Source: three-view drawing plus pictorial views. Frame: mm from the lowest corner of the part. A direction names the side the tool comes from. Give positions to 0.01 mm unless a question says otherwise; leave off trailing zeros. Loops run counter-clockwise (first coordinate to the right, second up) from the corner with the lowest first, then second, coordinate; pieces in that order, holes last. Notation, with made-up numbers: (-15, 6) - (7, 6) arc R29 cw to (7, 32) - close; hole circle Ø10 at (4, 45). An arc over 180 degrees is marked (long way). Put each result on its own line as item: value.
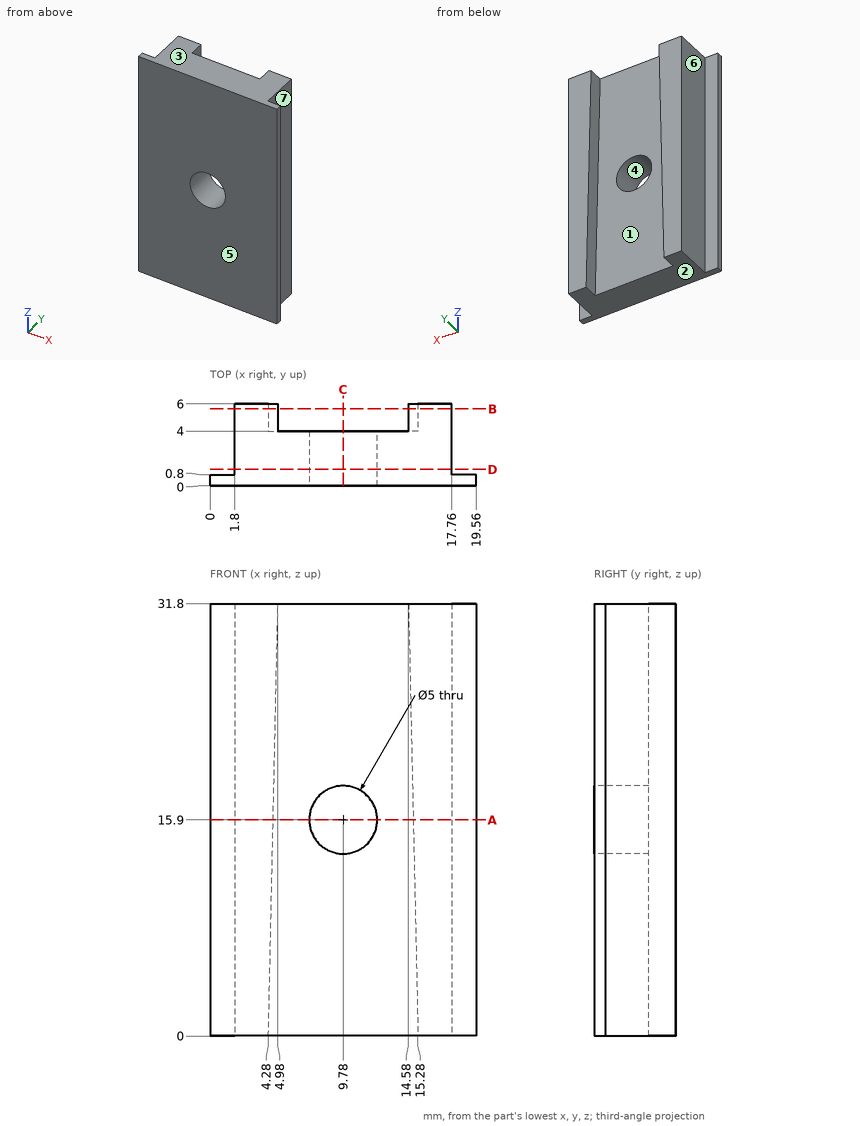
1) Section query B-B, the plane y = 5.65. Output: boundary loops of the cut face in (x, z), plus the area to 3 significant figures.
Check result:
outline: (1.8, 0) - (4.28, 0) - (4.98, 31.8) - (1.8, 31.8) - close; (14.58, 31.8) - (15.28, 0) - (17.76, 0) - (17.76, 31.8) - close
area: 180 mm²
2) Access query for the marked faces 5, 6 and 7. Directions: +Z, -Z, +X, -X, +Y, -Y. A direction counts if a zero-diameter tool reaches every point of the face in a straight line with its end or side. Return the directions, or none.
Check result:
face 5: +Z, -Z, +X, -X, -Y
face 6: +Z, -Z, -X, +Y
face 7: +Z, -Z, +X, +Y
3) Material intervals for line 1 along Z through (x, y) = (9.78, 1.5); line 2 along Y through (x, z) = (7.75, 22.5); line 3 along X through (y, z) = (0.9, 27.5), sorted ascending. Write a range as [from, to].
Check result:
line 1: [0, 13.4], [18.4, 31.8]
line 2: [0, 4]
line 3: [1.8, 17.76]
4) Mould query, pull axis Z, two halves, no side actions, for the marked faces 1, 2, 3 and 4. Classes: pulls with the +Z half, pulls with the -Z half, needs draft (parallel to the pull), parting line crosses it, or undercut.
Check result:
face 1: needs draft
face 2: pulls with the -Z half
face 3: pulls with the +Z half
face 4: undercut
5) Section query D-D, the plane y = 1.2. Output: boundary loops of the cut face in (x, z), plus the area to 3 significant figures.
Check result:
outline: (1.8, 0) - (17.76, 0) - (17.76, 31.8) - (1.8, 31.8) - close; hole circle Ø5 at (9.78, 15.9)
area: 488 mm²
6) Section query C-C, the plane x = 9.78. Output: boundary loops of the cut face in (y, z).
Check result:
outline: (0, 0) - (4, 0) - (4, 13.4) - (0, 13.4) - close; (0, 18.4) - (4, 18.4) - (4, 31.8) - (0, 31.8) - close
7) Pin query (flat end, axial travel): P1, Ø1.5, axis at y = 5, z = 23, coming from the -X side; P2, Ø1.4, axis at x = 0.5, z = 8.5, coming from the +Y side; P3, Ø5, axis at x = 12, z = 24.5, coming from the +Y side. Return the tip coordinate at first contact, or that it passes through.
Check result:
P1: x = 1.8
P2: y = 0.8
P3: y = 4
8) Section query A-A, the plane z = 15.9. Output: boundary loops of the cut face in (x, y), plus the area to 3 significant figures.
Check result:
outline: (0, 0) - (7.28, 0) - (7.28, 4) - (4.63, 4) - (4.63, 6) - (1.8, 6) - (1.8, 0.8) - (0, 0.8) - close; (12.28, 0) - (19.56, 0) - (19.56, 0.8) - (17.76, 0.8) - (17.76, 6) - (14.93, 6) - (14.93, 4) - (12.28, 4) - close
area: 58.0 mm²
